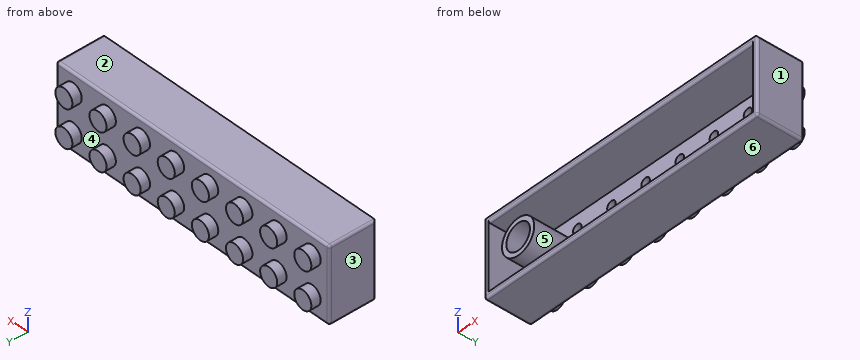
```python
from build123d import *

# Parameters (mm, degrees)
BOSS_EXTRUDE1_DEPTH      = 8
BOSS_EXTRUDE1_DEPTH_BACK = 8
SKETCH1_W                = 64
SKETCH1_H                = 10
SKETCH2_R                = 2
BOSS_EXTRUDE2_DEPTH      = 2
SHELL1_T                 = -1
SKETCH3_R                = 3.772610986
SKETCH3_R_2              = 2.772610986
BOSS_EXTRUDE3_DEPTH      = 9
FILLET1_R                = 0.5


with BuildPart() as part:
    # Sketch1 → Boss-Extrude1 (new, two sides: drawn at the far end of the back side and taken through both)
    with BuildSketch(Plane.XY.offset(-BOSS_EXTRUDE1_DEPTH_BACK)):
        Rectangle(SKETCH1_W, SKETCH1_H)
    extrude(amount=BOSS_EXTRUDE1_DEPTH + BOSS_EXTRUDE1_DEPTH_BACK)

    # Sketch2 → Boss-Extrude2 (add)
    with BuildSketch(Plane(origin=(0, 5, 0), x_dir=(1, 0, 0), z_dir=(0, 1, 0))):
        with Locations(Location((-28, 4, 0), (0, 0, 270))):
            Circle(SKETCH2_R)
        with Locations(Location((-20, 4, 0), (0, 0, 270))):
            Circle(SKETCH2_R)
        with Locations(Location((-12, 4, 0), (0, 0, 270))):
            Circle(SKETCH2_R)
        with Locations(Location((-4, 4, 0), (0, 0, 270))):
            Circle(SKETCH2_R)
        with Locations(Location((4, 4, 0), (0, 0, 270))):
            Circle(SKETCH2_R)
        with Locations(Location((12, 4, 0), (0, 0, 270))):
            Circle(SKETCH2_R)
        with Locations(Location((20, 4, 0), (0, 0, 270))):
            Circle(SKETCH2_R)
        with Locations(Location((28, 4, 0), (0, 0, 270))):
            Circle(SKETCH2_R)
        with Locations(Location((-20, -4, 0), (0, 0, 270))):
            Circle(SKETCH2_R)
        with Locations(Location((-12, -4, 0), (0, 0, 270))):
            Circle(SKETCH2_R)
        with Locations(Location((-4, -4, 0), (0, 0, 270))):
            Circle(SKETCH2_R)
        with Locations(Location((4, -4, 0), (0, 0, 270))):
            Circle(SKETCH2_R)
        with Locations(Location((12, -4, 0), (0, 0, 270))):
            Circle(SKETCH2_R)
        with Locations(Location((20, -4, 0), (0, 0, 270))):
            Circle(SKETCH2_R)
        with Locations(Location((28, -4, 0), (0, 0, 270))):
            Circle(SKETCH2_R)
        with Locations(Location((-28, -4, 0), (0, 0, 270))):
            Circle(SKETCH2_R)
    extrude(amount=BOSS_EXTRUDE2_DEPTH)

    # Shell1
    shell1_openings = [part.faces().sort_by_distance(p)[0] for p in [
        (0, -5, 0),
    ]]
    offset(amount=SHELL1_T, openings=shell1_openings, kind=Kind.INTERSECTION)

    # Sketch3 → Boss-Extrude3 (add)
    with BuildSketch(Plane(origin=(0, 4, 0), x_dir=(-1, 0, 0), z_dir=(0, -1, 0))):
        with Locations(Location((24, 0, 0), (0, 0, 270))):
            Circle(SKETCH3_R)
        with Locations(Location((24, 0, 0), (0, 0, 90))):
            Circle(SKETCH3_R_2, mode=Mode.SUBTRACT)
    extrude(amount=BOSS_EXTRUDE3_DEPTH)

    # Fillet1
    fillet1_edges = [part.edges().sort_by_distance(p)[0] for p in [
        (-32, 0, -8),
        (32, 0, 8),
        (0, 5, 8),
        (0, -5, -8),
        (-32, 0, 8),
        (32, 0, -8),
        (0, 5, -8),
        (32, -5, 0),
        (-32, -5, 0),
        (-32, 5, 0),
        (32, 5, 0),
        (0, -5, 7),
    ]]
    fillet(fillet1_edges, radius=FILLET1_R)


solid = part.part
```
Geometry: final body of the model. Coordinates: model frame, mm. Face numbers are marked on the shaded views. A direction names the side the tool comes from. Coordinates: 2 decimals unless noted, no trailing zeros. Write each loop counter-clockwise with the first axis right and the second up, starting at its lowest first coordinate (ties: lowest second). Pieces come first, ordered by that corner, then holes. Notation, with made-up numbers: M 50,13 L 55,13 A8 cw 55,26 Z; hole C 13,-14.5 d8. An arc over 180 degrees is marked long. Answer as CSV lines item,"result". Start each with the question number.
Q1. Cut plane B-B on x = -16.5. Return the cut outline in (y, z), then the cut area to 3 significant figures.
Q2. Reachability of the marked faces 5 and 6 from +Z, -Z, +X, -X, +Y, -Y: full face, straight path, thin tool, end or side. Return the list, or none.
Q3. Cut plane C-C on z = 0. Return the cut outline in (x, y), then the cut area to 3 significant figures.
Q4. Mould query, pull axis X, two halves, no side actions, for the marked faces 1, 2, 3 and 4. Classes: released by +X, released by -X, zero draft, split by the parting line, or undercut.
Q5. Line query: line 1 (Z direction, x = 4, y = 4.55); line 2 (Z direction, x = -10, y = -2.5); line 3 (X direction, y = -0.75, z = -6.5). Output: solid intervals per line, ascending. Write a range as from..to.
Q6. Cut plane A-A on y = -3. Return the cut outline in (x, z).
Q7. Pin query (flat end, axial travel): P1, Ø1.6, axis at x = -20, z = 4, coming from the -Y side; P2, Ø2.5, axis at x = -4, z = 4, coming from the -Y side; P3, Ø6, axis at x = -6.5, z = 3.5, coming from the +Y side. Return the tip coordinate at first contact, or that it passes through.
Findings below:
1,outline,"M -5,-7.5 A0.5 ccw -4.5,-8 L 4.5,-8 A0.5 ccw 5,-7.5 L 5,7.5 A0.5 ccw 4.5,8 L -5,8 L -5,7.5 A0.5 ccw -4.5,7 L 4,7 L 4,-7 L -5,-7 Z"
1,area,"33.8 mm2"
2,face 5,"-Y"
2,face 6,"-Z, +X, -X, +Y, -Y"
3,outline,"M -32,-4.5 A0.5 ccw -31.5,-5 L -31,-5 L -31,4 L -27.77,4 L -27.77,-5 L -26.77,-5 L -26.77,4 L -21.23,4 L -21.23,-5 L -20.23,-5 L -20.23,4 L 31,4 L 31,-5 L 31.5,-5 A0.5 ccw 32,-4.5 L 32,4.5 A0.5 ccw 31.5,5 L -31.5,5 A0.5 ccw -32,4.5 Z"
3,area,"99.8 mm2"
4,face 1,"released by +X"
4,face 2,"zero draft"
4,face 3,"released by -X"
4,face 4,"undercut"
5,line 1,"z = -8..-5, -3..3, 5..8"
5,line 2,"z = -8..-7, 7..8"
5,line 3,"x = -32..-31, 31..32"
6,outline,"M -32,-7.5 A0.5 ccw -31.5,-8 L 31.5,-8 A0.5 ccw 32,-7.5 L 32,7.5 A0.5 ccw 31.5,8 L -31.5,8 A0.5 ccw -32,7.5 Z; C -24,0 d7.55; hole M -31,-7 L 31,-7 L 31,7 L -31,7 Z; hole C -24,0 d5.55"
7,P1,"stops at y = 6"
7,P2,"stops at y = 4"
7,P3,"stops at y = 7"
